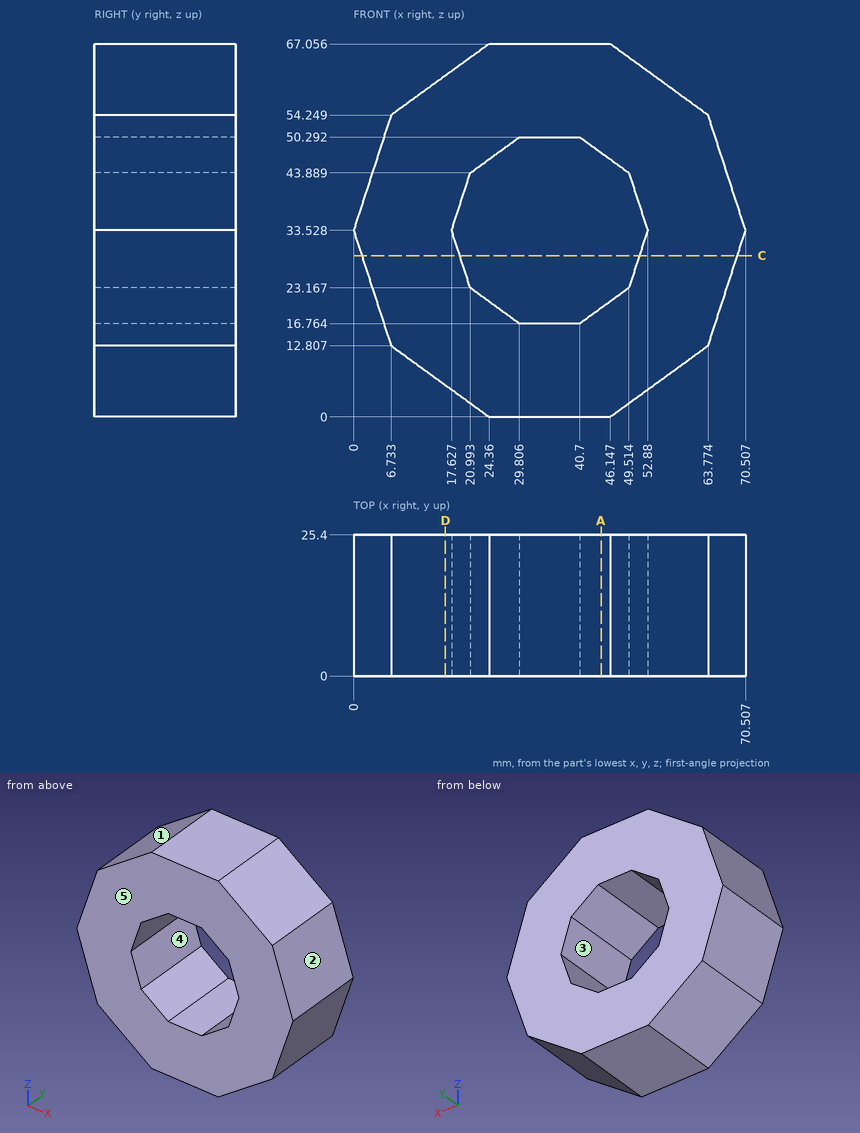
Job drawing, mm, ordinate dimensions from the low corner. One solid piece. A direction names the side the tool comes from. Round coordinates to 2 decimals unless told otherwise and drop trailing zeros. Loops run counter-clockwise (first coordinate to the right, second up) from the corner with the lowest first, then second, coordinate; pieces in that order, holes last. Notation, with made-up numbers: M 7,86.25 L 27,86.25 A30 cw 27,123.25 Z; hole C -18.75,-7.75 d5. An arc over 180 degrees is marked long. Answer as CSV lines item,"result".
1. 3-axis set-ups, long thin cutter, end or side, ignore diameter. For the marked faces 4 and 5: which of +Z, -Z, +X, -X, +Y, -Y reach the whole face in a straight line?
Resolved:
face 4,"+Y, -Y"
face 5,"+Z, -Z, +X, -X, -Y"
2. Cut at C-C on z = 29. Write the cut outline in (x, y) (1 decimal).
Resolved:
outline,"M 1.5,0 L 19.1,0 L 19.1,25.4 L 1.5,25.4 Z; M 51.4,0 L 69,0 L 69,25.4 L 51.4,25.4 Z"
3. Wall check: probe 1 along Z at (x, y) = (30, 18.5); probe 2 along Z at (x, y) = (49, 1.75) (1 decimal); probe 3 along X at (y, z) = (14.75, 41.5) (1 decimal). Give the ranges that are in metal, low to high. Write a range as [from, to].
Resolved:
probe 1,"z = [0, 16.76], [50.29, 67.06]"
probe 2,"z = [2.1, 22.8], [44.3, 65]"
probe 3,"x = [2.6, 20.2], [50.3, 67.9]"
4. Two-plate mould, pull along X, no slides. Class the marked faces 1, 2 and 3: released by +X, released by -X, zero draft, split by the parting line, or undercut.
Resolved:
face 1,"released by -X"
face 2,"released by +X"
face 3,"undercut"
5. Cut at D-D on x = 16.5. Write the cut outline in (y, z) (1 decimal).
Resolved:
outline,"M 0,5.7 L 25.4,5.7 L 25.4,61.3 L 0,61.3 Z"
6. Cut at A-A on x = 44.5. Write the cut outline in (y, z) (1 decimal), then the cut area to 3 significant figures.
Resolved:
outline,"M 0,0 L 25.4,0 L 25.4,19.5 L 0,19.5 Z; M 0,47.5 L 25.4,47.5 L 25.4,67.1 L 0,67.1 Z"
area,"992 mm²"
7. Flat gauge pins, fed straight in: P1, Ø1, axis at y = 17.5, z = 53.5, coming from the -X side; P2, Ø4, axis at y = 13, z = 21, coming from the +X side; P3, Ø4, axis at x = 8.5, y = 4, coming from the +Z side (1 decimal). Where does each tip first touch, or does it go through?
Resolved:
P1,"stops at x = 6.33"
P2,"stops at x = 67.09"
P3,"stops at z = 57"
